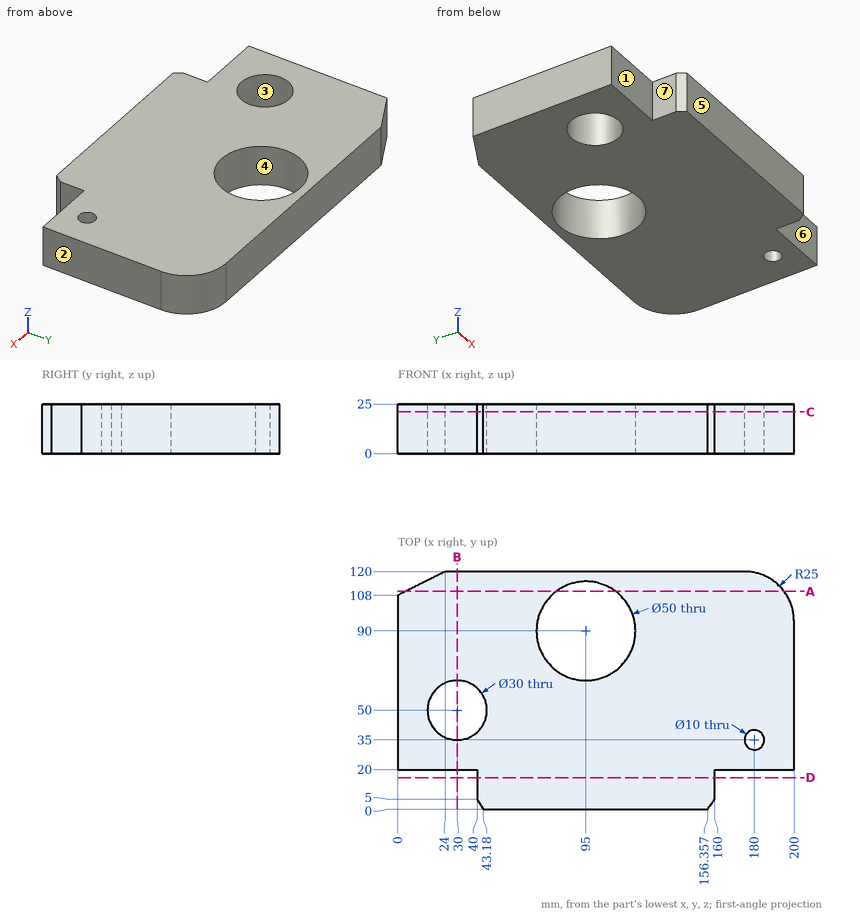
Study the drawing (mm; zero at the part's minimum x, y, z) and answer. A direction names the side the tool comes from. Give positions to 0.01 mm unless a question says otherwise; leave off trailing zeros. Loops run counter-clockwise (first coordinate to the right, second up) from the corner with the lowest first, then second, coordinate; pieces in that order, holes last. Notation, with made-up numbers: (-9, 26.25) - (34, 26.25) arc R10 cw to (34, 42.25) - close; hole circle Ø1 at (33, -16). An arc over 180 degrees is marked (long way). Answer as CSV lines item,"result". Start each with the question number.
1) Find section A-A (y = 110). Write down the section's boundary in (x, z), then the cut area to 4 significant figures.
2) Each of these flat-tipped pins is pushed along its axis until it touches: pin 1 Ø4.5 at (y, z) = (9, 9.5) entering from -X; pin 2 Ø4.5 at (y, z) = (12, 18.5) entering from +X; pin 3 Ø4 at (x, z) = (35.5, 17.5) entering from -Y. Where does it stop, or does it pass through?
3) Find section D-D (y = 16). Write down the section's boundary in (x, z).
4) Which of the six approach directions +Z, -Z, +X, -X, +Y, -Y give full straight-line access (tool end or side, diameter ignored) to the marked faces 5, 6 and 7?
5) Find section B-B (x = 30). Write down the section's boundary in (y, z), then the cut area to 3 significant figures.
6) Find section C-C (z = 21). Write down the section's boundary in (x, y).
7) Determine the mould class of the marked faces 1, 2, 3 and 4 for opening direction X: released by +X, released by -X, zero draft, split by the parting line, or undercut.
8) Straight lines are drawn through the part: L1, parallel to Y at x = 95, z = 5.5; L2, parallel to X at y = 51, z = 14; L3, parallel to Y at x = 30, z = 16.25. For each, find the intervals that lie inside material, in ascending order. Write a range as from..to.
Findings below:
1,outline,"(4, 0) - (80, 0) - (80, 25) - (4, 25) - close; (110, 0) - (195, 0) - (195, 25) - (110, 25) - close"
1,area,"4,025 mm^2"
2,pin 1,"x = 40"
2,pin 2,"x = 160"
2,pin 3,"y = 20"
3,outline,"(40, 0) - (160, 0) - (160, 25) - (40, 25) - close"
4,face 5,"+Z, -Z, +X, -X, -Y"
4,face 6,"+Z, -Z, +X, -Y"
4,face 7,"+Z, -Z, -X, -Y"
5,outline,"(20, 0) - (35, 0) - (35, 25) - (20, 25) - close; (65, 0) - (120, 0) - (120, 25) - (65, 25) - close"
5,area,"1,750 mm^2"
6,outline,"(0, 20) - (40, 20) - (40, 5) - (43.18, 0) - (156.36, 0) - (160, 5) - (160, 20) - (200, 20) - (200, 95) arc R25 ccw to (175, 120) - (24, 120) - (0, 108) - close; hole circle Ø30 at (30, 50); hole circle Ø50 at (95, 90); hole circle Ø10 at (180, 35)"
7,face 1,"zero draft"
7,face 2,"released by +X"
7,face 3,"undercut"
7,face 4,"undercut"
8,L1,"0..65, 115..120"
8,L2,"0..15.03, 44.97..200"
8,L3,"20..35, 65..120"
